Part model, mm, in its own coordinate system. A direction names the side the tool comes from. Give positions to 0.01 mm unless a question says otherwise; leave off trailing zeros. Write each loop counter-clockwise with the first axis right and the second up, starting at its lowest first coordinate (ties: lowest second). Pieces come first, ordered by that corner, then holes. Notation, with made-up numbers: (46, -32) - (103, -32) arc R29 ccw to (103, -4) - close; hole circle Ø11 at (24, 87.25). An arc over 180 degrees is marked (long way). Answer as a JSON object with one key per item and string values. Group by question number.
```python
from build123d import *

# Parameters (mm, degrees)
F1_DEPTH = 25.4
F2_R     = 9.525
F3_DEPTH = 66.676
F4_DEPTH = 66.676


with BuildPart() as f1:
    # F0 (on Top) → F1 (new body)
    with BuildSketch(Plane.XY):
        with BuildLine():
            Line((-60.410346, 74.541754), (-66.675, 73.258158))
            Line((-66.675, 73.258158), (-58.185558, -27.986543))
            ThreePointArc((-58.185558, -27.986543), (0, -66.056425), (58.185558, -27.986543))
            Line((58.185558, -27.986543), (66.675, 73.258158))
            Line((66.675, 73.258158), (60.388141, 74.276935))
            Line((60.388141, 74.276935), (55.189879, 12.282703))
            ThreePointArc((55.189879, 12.282703), (0, -59.706425), (-55.189879, 12.282703))
            Line((-55.189879, 12.282703), (-60.410346, 74.541754))
        make_face()
    extrude(amount=-F1_DEPTH)

    # F2 (on Right) → F3 (cut, through all)
    with BuildSketch(Plane.YZ):
        with Locations((58.328964, -13.568129)):
            Circle(F2_R)
    extrude(amount=F3_DEPTH, mode=Mode.SUBTRACT)

    # F2 (on Right) → F4 (cut, through all)
    with BuildSketch(Plane.YZ):
        with Locations((58.328964, -13.568129)):
            Circle(F2_R)
    extrude(amount=-F4_DEPTH, mode=Mode.SUBTRACT)


solid = f1.part
```
1) Mould opens along Z. For faces 1 (the flat face through (63.58, 73.76, -12.52)), 2 (the cylindrical face through (62.1, 50.8, -19.4)), 3 (the flat face through (15, -58, 0)), 4 (the cylindrical face through (-62.1, 50.8, -19.4)) say: pulls with the +Z half, pulls with the -Z half, needs draft (parallel to the pull), parting line crosses it, or undercut.
2) Band-saw the part on C-C (x = 0). List the corners of the cut face in (y, z), plus the area to 3 significant figures.
3) Probe line 1 (X direction, y = 33, z = -11.25); line 2 (X direction, y = 34, z = -8.75); line 3 (Y direction, x = 27, z = -6.75). List the from-to ranges inside material, lowest first.
4) Band-saw the part on A-A (z = -8). List the corners of the cut face in (x, y) (3 decimals), plus the area to 3 significant figures.
5) Band-saw the part on D-D (z = -16.5). List the corners of the cut face in (x, y) (3 decimals), plus the area to 3 significant figures.
6) Which spindle directions (+Z, -Z, +X, -X, +Y, -Y) get a long thin tool onto all of the face, cutting with end or side? Do faces 5 (the flat face through (62.37, 21.93, -12.52)), 6 (the flat face through (57.825, 43.714, -12.522)). Say none if no direction does.
7) Band-saw the part on B-B (y = 3.5). List the corners of the cut face in (x, z).
8) Drop flat-ended pins along their axis: P1, Ø3, axis at x = 32.5, z = -17.5, coming from the +Y side; P2, Ø2, axis at x = 23.5, z = -10, coming from the +Y side; P3, Ø2, axis at x = -27, z = -7.5, coming from the +Y side. Give the stop position or say it passes through.
Verdict:
{
 "1": {"face 1": "needs draft", "face 2": "undercut", "face 3": "pulls with the +Z half", "face 4": "undercut"},
 "2": {"outline": "(-66.06, -25.4) - (-59.71, -25.4) - (-59.71, 0) - (-66.06, 0) - close", "area": "161 mm2"},
 "3": {"line 1": "-63.3 to -56.93, 56.93 to 63.3", "line 2": "-63.38 to -57.01, 57.01 to 63.38", "line 3": "-60.03 to -52.93"},
 "4": {"outline": "(-66.675, 73.258) - (-66.071, 66.057) - (-59.699, 66.057) - (-60.41, 74.542) - close; (-64.775, 50.601) - (-58.186, -27.987) arc R63.5 ccw to (58.186, -27.987) - (64.775, 50.601) - (58.403, 50.601) - (55.19, 12.283) arc R57.15 cw (long way) to (-55.19, 12.283) - (-58.403, 50.601) - close; (59.699, 66.057) - (66.071, 66.057) - (66.675, 73.258) - (60.388, 74.277) - close", "area": "1,800 mm2"},
 "5": {"outline": "(-66.675, 73.258) - (-66.183, 67.392) - (-59.811, 67.392) - (-60.41, 74.542) - close; (-64.663, 49.266) - (-58.186, -27.987) arc R63.5 ccw to (58.186, -27.987) - (64.663, 49.266) - (58.291, 49.266) - (55.19, 12.283) arc R57.15 cw (long way) to (-55.19, 12.283) - (-58.291, 49.266) - close; (59.811, 67.392) - (66.183, 67.392) - (66.675, 73.258) - (60.388, 74.277) - close", "area": "1,760 mm2"},
 "6": {"face 5": "+Z, -Z, +X, -Y", "face 6": "+Z, -Z, +Y"},
 "7": {"outline": "(-60.83, -25.4) - (-56.83, -25.4) - (-56.83, 0) - (-60.83, 0) - close; (56.83, -25.4) - (60.83, -25.4) - (60.83, 0) - (56.83, 0) - close"},
 "8": {"P1": "y = -48.49", "P2": "y = -54.19", "P3": "y = -52.38"}
}
